Verification items for the finished model (mm, model axes). Face numbers are marked on the shaded views. A direction names the side the tool comes from. Round coordinates to 2 decimals unless told otherwise and drop trailing zeros. Loops run counter-clockwise (first coordinate to the right, second up) from the corner with the lowest first, then second, coordinate; pieces in that order, holes last. Notation, with made-up numbers: M -13.75,20 L 27.25,20 A27 ccw 27.25,36 Z; hole C 18,78.25 d3. An arc over 180 degrees is marked long. One line per item, written item: value.
from build123d import *

# Parameters (mm, degrees)
SKETCH1_R           = 15
SKETCH1_R_2         = 7.5
BOSS_EXTRUDE1_DEPTH = 85
SKETCH2_W           = 61
SKETCH2_H           = 50.965296902
CUT_EXTRUDE1_DEPTH  = 71
SKETCH3_R           = 10
CUT_EXTRUDE2_DEPTH  = 23


with BuildPart() as part:
    # Sketch1 → Boss-Extrude1 (new body)
    # profile 1 of 2: a face of its own
    with BuildSketch(Plane.XY):
        with BuildLine():
            Line((0, 15), (0, 0))
            Line((0, 0), (50, 0))
            Line((50, 0), (50, 15))
            Line((50, 15), (39.480230589, 53.914450421))
            ThreePointArc((39.480230589, 53.914450421), (39.869489884, 51.974403855), (40, 50))
            ThreePointArc((40, 50), (23.025596145, 35.130510116), (10.519769411, 53.914450421))
            Line((10.519769411, 53.914450421), (0, 15))
        make_face()
    # profile 2 of 2: a face of its own
    with BuildSketch(Plane.XY):
        with Locations((25, 50)):
            Circle(SKETCH1_R)
        with Locations((25, 50)):
            Circle(SKETCH1_R_2, mode=Mode.SUBTRACT)
    extrude(amount=-BOSS_EXTRUDE1_DEPTH)

    # Sketch2 → Cut-Extrude1 (cut)
    with BuildSketch(Plane(origin=(0, 0, 0), x_dir=(0, 0, -1), z_dir=(1, 0, 0))):
        with Locations((42.5, 40.482648451)):
            Rectangle(SKETCH2_W, SKETCH2_H)
    extrude(amount=CUT_EXTRUDE1_DEPTH, mode=Mode.SUBTRACT)

    # Sketch3 → Cut-Extrude2 (cut)
    with BuildSketch(Plane(origin=(0, 15, 0), x_dir=(1, 0, 0), z_dir=(0, 1, 0))):
        with Locations(Location((25, 42.5, 0), (0, 0, 270))):
            Circle(SKETCH3_R)
    extrude(amount=-CUT_EXTRUDE2_DEPTH, mode=Mode.SUBTRACT)


solid = part.part
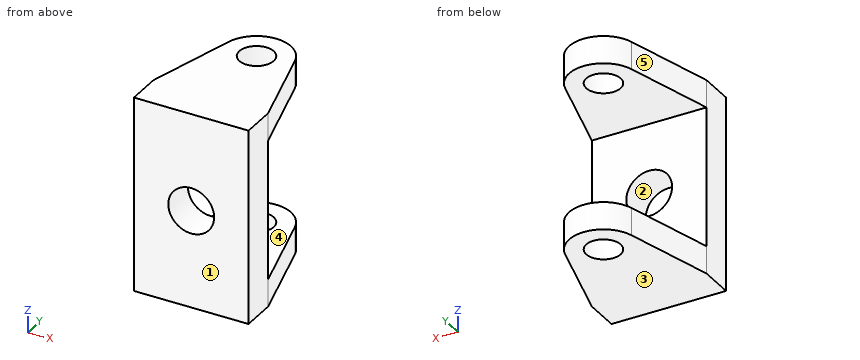
(1) Sectioned sample at D-D on y = 16. Enter the section's corners in (x, z), and give its area (3 significant figures).
Completed:
outline: M 0.27,-85 L 49.73,-85 L 49.73,-73 L 0.27,-73 Z; M 0.27,-12 L 49.73,-12 L 49.73,0 L 0.27,0 Z
area: 1,190 mm^2
(2) Sectioned sample at C-C on z = -7.5. Enter the section's corners in (x, y), and give its area (3 significant figures).
Completed:
outline: M 0,0 L 50,0 L 50,15 L 39.48,53.91 A15 ccw 10.52,53.91 L 0,15 Z; hole C 25,50 d15
area: 2,350 mm^2
(3) Sectioned sample at B-B on z = -42.5. Enter the section's corners in (x, y).
Completed:
outline: M 0,0 L 15,0 L 15,15 L 0,15 Z; M 35,0 L 50,0 L 50,15 L 35,15 Z
(4) Mould release check, pull along Z, two halves, no side actions. Record for the marked faces 1, 2 and 3: +Z half, -Z half, draft (parallel to the pull), parting line (faces both ways), or undercut.
Completed:
face 1: draft
face 2: undercut
face 3: -Z half
(5) Tool access check on the marked faces 4 and 5. Record the directions out of +Z, -Z, +X, -X, +Y, -Y that give a thin tool (end or side, any length) a straight path to the whole face; none if there is none.
Completed:
face 4: +X, -X, +Y
face 5: +Z, -Z, -X, +Y
(6) Depth check by flat-ended pin: pin 1 Ø15 at (x, z) = (24.5, -50) entering from +Y. Enter the tip coordinate at first touch or a pass-through.
Completed:
pin 1: stops at y = 15
(7) Thickness scan on L1, parallel to Z at x = 43, y = 31.5; L2, parallel to Y at x = 15, z = -28.5; L3, parallel to Z at x = 21, y = 11. Record the ranges inside material, lowest first. Write a range as from..to.
Completed:
L1: z = -85..-73, -12..0
L2: y = 0..15
L3: z = -85..-51.67, -33.33..0
(8) Sectioned sample at A-A on x = 25. Enter the section's corners in (y, z).
Completed:
outline: M 0,-85 L 42.5,-85 L 42.5,-73 L 15,-73 L 15,-52.5 L 0,-52.5 Z; M 0,-32.5 L 15,-32.5 L 15,-12 L 42.5,-12 L 42.5,0 L 0,0 Z; M 57.5,-85 L 65,-85 L 65,-73 L 57.5,-73 Z; M 57.5,-12 L 65,-12 L 65,0 L 57.5,0 Z
